Geometry: final body of the model. Coordinates: model frame, mm. Face numbers are marked on the shaded views. A direction names the side the tool comes from. Round coordinates to 2 decimals unless told otherwise and drop trailing zeros. Write each loop counter-clockwise with the first axis right and the second up, starting at its lowest first coordinate (ties: lowest second). Pieces come first, ordered by that corner, then holes. Notation, with made-up numbers: (50, 50.5) -> (90, 50.5) arc R22 cw to (90, 83.5) -> close; hole circle Ø10 at (-37.5, 63). An arc over 180 degrees is marked (long way). Use one line per item in the form item = value. Start each with the question number.
1. Cut plane C-C, the plane x = 68. Return the cut outline in (y, z).
2. Cut plane A-A, the plane z = -34. Return the cut outline in (x, y).
3. Cut plane B-B, the plane z = -17. Return the cut outline in (x, y).
4. Reachability of the marked faces 1, 2 and 3 from +Z, -Z, +X, -X, +Y, -Y: full face, straight path, thin tool, end or side. Return the list, or none.
5. Cut plane D-D, the plane y = 5.75. State how many separate pieces and enclosed holes the cut face has, plus the area to 3 significant figures.
6. Line query: L1, parallel to X at y = 12, z = -4; L2, parallel to X at y = 10.5, z = -17; L3, parallel to X at y = 14, z = -9. Output: solid intervals per line, ascending.
7. Draft query along Z for the marked faces 4, 5, 6 and 7. Return one class per face: pulls with the +Z half, pulls with the -Z half, needs draft (parallel to the pull), parting line crosses it, or undercut.
8. Pin query (flat end, axial travel): pin 1 Ø8 at (x, y) = (52.5, 7) entering from +Z; pin 2 Ø10 at (y, z) = (6.5, -19) entering from +X; pin 3 Ø6 at (x, y) = (43, 17.5) entering from -Z. Return the tip coordinate at first contact, or that it passes through.
```python
from build123d import *

# Parameters (mm, degrees)
BOSS_EXTRUDE2_DEPTH = 20
CUT_EXTRUDE1_DEPTH  = 21


with BuildPart() as part:
    # Sketch1 → Boss-Extrude2 (new body)
    with BuildSketch(Plane(origin=(0, 0, 0), x_dir=(1, 0, 0), z_dir=(0, 1, 0))):
        Polygon((21, -13.279056191), (21, -19.052558883), (23, -19.052558883), (23, -13.279056191), (33, -7.505553499), (43, -13.279056191), (43, -19.052558883), (45, -19.052558883), (45, -13.279056191), (55, -7.505553499), (65, -13.279056191), (65, -19.052558883), (67, -19.052558883), (67, -13.279056191), (77, -7.505553499), (77, 7.400435733), (67, 13.173938425), (67, 24.720943809), (77, 30.494446501), (77, 38), (76, 38), (76, 32.226497308), (66, 26.452994616), (56, 32.226497308), (56, 38), (54, 38), (54, 32.226497308), (44, 26.452994616), (34, 32.226497308), (34, 38), (32, 38), (32, 32.226497308), (22, 26.452994616), (12, 32.226497308), (12, 38), (11, 38), (11, 30.494446501), (21, 24.720943809), (21, 13.173938425), (11, 7.400435733), (11, -7.505553499), align=None)
        Polygon((12, 5.773502692), (22, 11.547005384), (32, 5.773502692), (32, -5.773502692), (22, -11.547005384), (12, -5.773502692), align=None, mode=Mode.SUBTRACT)
        Polygon((34, 5.773502692), (44, 11.547005384), (54, 5.773502692), (54, -5.773502692), (44, -11.547005384), (34, -5.773502692), align=None, mode=Mode.SUBTRACT)
        Polygon((56, 5.773502692), (66, 11.547005384), (76, 5.773502692), (76, -5.773502692), (66, -11.547005384), (56, -5.773502692), align=None, mode=Mode.SUBTRACT)
        Polygon((43, 13.173938425), (33, 7.400435733), (23, 13.173938425), (23, 24.720943809), (33, 30.494446501), (43, 24.720943809), align=None, mode=Mode.SUBTRACT)
        Polygon((65, 13.173938425), (55, 7.400435733), (45, 13.173938425), (45, 24.720943809), (55, 30.494446501), (65, 24.720943809), align=None, mode=Mode.SUBTRACT)
    extrude(amount=BOSS_EXTRUDE2_DEPTH)

    # Sketch2 → Cut-Extrude1 (cut, through all)
    with BuildSketch(Plane(origin=(0, 20, 0), x_dir=(1, 0, 0), z_dir=(0, 1, 0))):
        Polygon((11, 6.245735195), (22, 12.596588156), (22, 25.298294078), (11, 31.649147039), (2.295872016, -19.052558883), (22, -19.052558883), (22, -12.701705922), (11, -6.350852961), align=None)
        Polygon((77, 31.649147039), (85.704127984, -19.052558883), (66, -19.052558883), (66, -12.701705922), (77, -6.350852961), (77, 6.245735195), (66, 12.596588156), (66, 25.298294078), align=None)
    extrude(amount=-CUT_EXTRUDE1_DEPTH, mode=Mode.SUBTRACT)


solid = part.part
```
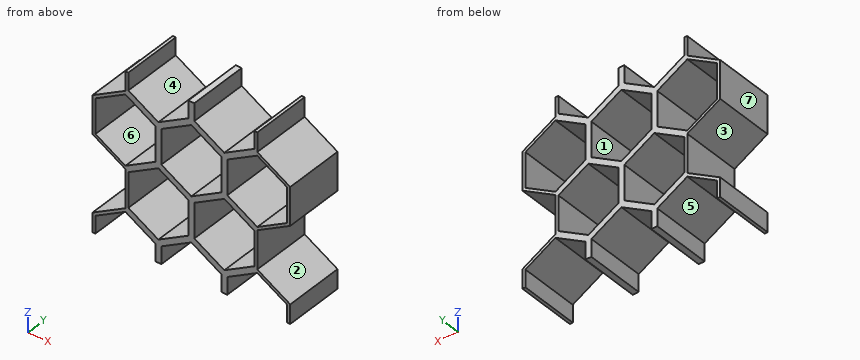
Outcome:
q1.outline = (0, -27.61) -> (20, -27.61) -> (20, -26.45) -> (0, -26.45) -> close; (0, -11.44) -> (20, -11.44) -> (20, -10.39) -> (0, -10.39) -> close; (0, 10.39) -> (20, 10.39) -> (20, 11.55) -> (0, 11.55) -> close
q2.outline = (11, 0) -> (12, 0) -> (12, 20) -> (11, 20) -> close; (32, 0) -> (34, 0) -> (34, 20) -> (32, 20) -> close; (54, 0) -> (56, 0) -> (56, 20) -> (54, 20) -> close; (76, 0) -> (77, 0) -> (77, 20) -> (76, 20) -> close
q3.outline = (22, 0) -> (23, 0) -> (23, 20) -> (22, 20) -> close; (43, 0) -> (45, 0) -> (45, 20) -> (43, 20) -> close; (65, 0) -> (66, 0) -> (66, 20) -> (65, 20) -> close
q4.face_1 = +Y, -Y
q4.face_2 = +X, +Y, -Y
q4.face_3 = -X, +Y, -Y
q5.separate_pieces = 1
q5.enclosed_holes = 5
q5.area = 539 mm^2
q6.L1 = 11 to 12, 32 to 34, 54 to 56, 76 to 77
q6.L2 = 22 to 23, 43 to 45, 65 to 66
q6.L3 = 15.77 to 17.59, 26.41 to 30.23, 35.77 to 39.59, 48.41 to 52.23, 57.77 to 61.59, 70.41 to 72.23
q7.face_4 = pulls with the +Z half
q7.face_5 = pulls with the -Z half
q7.face_6 = undercut
q7.face_7 = needs draft
q8.pin_1 = 11.26
q8.pin_2 = 66
q8.pin_3 = -28.76
